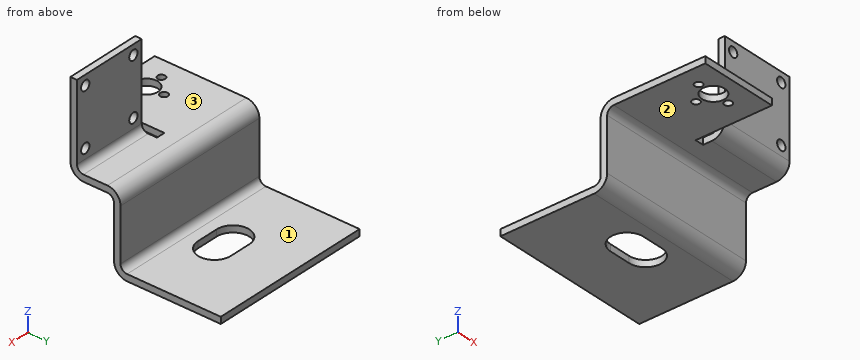
from build123d import *

# Parameters (mm, degrees)
SKETCH1_W                    = 35
SKETCH1_H                    = 35
SKETCH1_R                    = 2.25
BASE_FLANGE1_DEPTH           = 3
EDGE_FLANGE1_DEPTH           = 35
SKETCH9_W                    = 36
SKETCH9_H                    = 35
BOSS_EXTRUDE1_DEPTH          = 3
EDGE_FLANGE2_STRIP_W         = 18
EDGE_FLANGE2_STRIP_H         = 3
EDGE_FLANGE2_STRIP_CUT_DEPTH = 75
EDGE_FLANGE2_DEPTH           = 75
EDGE_FLANGE3_STRIP_W         = 18
EDGE_FLANGE3_STRIP_H         = 3
EDGE_FLANGE3_STRIP_CUT_DEPTH = 75
EDGE_FLANGE3_DEPTH           = 75
SKETCH16_R                   = 5.25
SKETCH16_R_2                 = 1.75
CUT_EXTRUDE1_DEPTH           = 10
CUT_EXTRUDE2_DEPTH           = 10
BODY_MOVE_COPY1_ANGLE        = 180


# Sheet-metal steps are written as plain solids
with BuildPart() as part:
    # Sketch1 → Base-Flange1 (new body)
    with BuildSketch(Plane.XY):
        Rectangle(SKETCH1_W, SKETCH1_H)
        with Locations((-13, 13)):
            Circle(SKETCH1_R, mode=Mode.SUBTRACT)
        with Locations((13, 13)):
            Circle(SKETCH1_R, mode=Mode.SUBTRACT)
        with Locations((13, -13)):
            Circle(SKETCH1_R, mode=Mode.SUBTRACT)
        with Locations((-13, -13)):
            Circle(SKETCH1_R, mode=Mode.SUBTRACT)
    extrude(amount=-BASE_FLANGE1_DEPTH)

    # Edge-Flange1 section (across the edge) → Edge-Flange1 (add)
    with BuildSketch(Plane(origin=(-17.5, -20.5, 0), x_dir=(0, 1, 0), z_dir=(1, 0, 0))):
        with BuildLine():
            Line((-3, 3), (-3, 17))
            Line((-3, 17), (0, 17))
            Line((0, 17), (0, 3))
            ThreePointArc((0, 3), (0.878679656, 0.878679656), (3, 0))
            Line((3, 0), (3, -3))
            ThreePointArc((3, -3), (-1.242640687, -1.242640687), (-3, 3))
        make_face()
    extrude(amount=EDGE_FLANGE1_DEPTH)

    # Sketch9 → Boss-Extrude1 (add)
    with BuildSketch(Plane.XZ.offset(23.5)):
        Polygon((57.5, 17), (17.5, 17), (17.5, 7), (21.5, 7), (57.5, 7), align=None)
        with Locations((39.5, -10.5)):
            Rectangle(SKETCH9_W, SKETCH9_H)
    extrude(amount=-BOSS_EXTRUDE1_DEPTH)

    # Edge-Flange2 strip (across the edge) → Edge-Flange2 strip cut (cut)
    with BuildSketch(Plane(origin=(57.5, -23.5, 17), x_dir=(0, 0, -1), z_dir=(-1, 0, 0))):
        with Locations((-6, -1.5)):
            Rectangle(EDGE_FLANGE2_STRIP_W, EDGE_FLANGE2_STRIP_H)
    extrude(amount=EDGE_FLANGE2_STRIP_CUT_DEPTH, mode=Mode.SUBTRACT)

    # Edge-Flange2 section (across the edge) → Edge-Flange2 (add)
    with BuildSketch(Plane(origin=(57.5, -23.5, 17), x_dir=(0, 0, -1), z_dir=(-1, 0, 0))):
        with BuildLine():
            Line((-3, 3), (-3, 30))
            Line((-3, 30), (0, 30))
            Line((0, 30), (0, 3))
            ThreePointArc((0, 3), (0.878679656, 0.878679656), (3, 0))
            Line((3, 0), (3, -3))
            ThreePointArc((3, -3), (-1.242640687, -1.242640687), (-3, 3))
        make_face()
    extrude(amount=EDGE_FLANGE2_DEPTH)

    # Edge-Flange3 strip (across the edge) → Edge-Flange3 strip cut (cut)
    with BuildSketch(Plane(origin=(-17.5, -53.5, 20), x_dir=(0, 1, 0), z_dir=(1, 0, 0))):
        with Locations((-6, -1.5)):
            Rectangle(EDGE_FLANGE3_STRIP_W, EDGE_FLANGE3_STRIP_H)
    extrude(amount=EDGE_FLANGE3_STRIP_CUT_DEPTH, mode=Mode.SUBTRACT)

    # Edge-Flange3 section (across the edge) → Edge-Flange3 (add)
    with BuildSketch(Plane(origin=(-17.5, -53.5, 20), x_dir=(0, 1, 0), z_dir=(1, 0, 0))):
        with BuildLine():
            Line((-3, 3), (-3, 46))
            Line((-3, 46), (0, 46))
            Line((0, 46), (0, 3))
            ThreePointArc((0, 3), (0.878679656, 0.878679656), (3, 0))
            Line((3, 0), (3, -3))
            ThreePointArc((3, -3), (-1.242640687, -1.242640687), (-3, 3))
        make_face()
    extrude(amount=EDGE_FLANGE3_DEPTH)

    # Sketch16 → Cut-Extrude1 (cut)
    with BuildSketch(Plane(origin=(0, -20.5, 0), x_dir=(1, 0, 0), z_dir=(0, 1, 0))):
        with Locations(Location((40.5, 17.3, 0), (0, 0, 270))):
            Circle(SKETCH16_R)
        with Locations(Location((40.5, 9.3, 0), (0, 0, 270))):
            Circle(SKETCH16_R_2)
        with Locations(Location((48.5, 17.3, 0), (0, 0, 270))):
            Circle(SKETCH16_R_2)
        with Locations(Location((32.5, 17.3, 0), (0, 0, 270))):
            Circle(SKETCH16_R_2)
    extrude(amount=-CUT_EXTRUDE1_DEPTH, mode=Mode.SUBTRACT)

    # Sketch17 → Cut-Extrude2 (cut)
    with BuildSketch(Plane(origin=(0, -53.5, 0), x_dir=(1, 0, 0), z_dir=(0, 1, 0))):
        with BuildLine():
            Line((25, -43), (15, -43))
            ThreePointArc((15, -43), (7.5, -35.5), (15, -28))
            Line((15, -28), (25, -28))
            ThreePointArc((25, -28), (32.5, -35.5), (25, -43))
        make_face()
    extrude(amount=-CUT_EXTRUDE2_DEPTH, mode=Mode.SUBTRACT)


with BuildPart() as part_1:
    # Body-Move/Copy1: moved
    add(part.part.moved(Location((0, 0, 0))).rotate(Axis((20, -19.25, 19.25), (-4.937700262163626e-15, 0.7071067811864181, 0.707106781186677)), BODY_MOVE_COPY1_ANGLE))


solid = part_1.part
Design review of the part built by this model. Coordinates are the model's own, in mm. Face numbers are marked on the shaded views. A direction names the side the tool comes from. Give positions to 0.01 mm unless a question says otherwise; leave off trailing zeros. Order: outer loops, then holes, each group sorted by start corner. A loop starts at its lowest first (then second) coordinate and runs counter-clockwise, first axis right, second up.
1. Tool access review of the marked faces 1, 2 and 3: name each direction out of +Z, -Z, +X, -X, +Y, -Y from which nothing blocks a thin tool from reaching the whole face with its end or side.
Solution:
face 1: +Z, +X, -X, +Y
face 2: -Z, +X, -X, -Y
face 3: +Z, -X, +Y
2. Add section D-D, the plane x = -8.5. State the section outline as (y, z) points, then the cut area to 3 significant figures.
Solution:
outline: (-66.5, 15) - (-57.55, 15) - (-57.55, 18) - (-66.5, 18) - close; (-54.05, 15) - (-24.5, 15) arc R3 cw to (-21.5, 12) - (-21.5, -12) arc R6 ccw to (-15.5, -18) - (27.5, -18) - (27.5, -15) - (-15.5, -15) arc R3 cw to (-18.5, -12) - (-18.5, 12) arc R6 ccw to (-24.5, 18) - (-54.05, 18) - close
area: 359 mm2
3. Add section B-B, the plane z = 51.5. State the section outline as (x, y) points.
Solution:
outline: (22.5, -41.5) - (24.75, -41.5) - (24.75, -38.5) - (22.5, -38.5) - close; (29.25, -41.5) - (50.75, -41.5) - (50.75, -38.5) - (29.25, -38.5) - close; (55.25, -41.5) - (57.5, -41.5) - (57.5, -38.5) - (55.25, -38.5) - close
4. Add section C-C, the plane y = -47.8. State the section outline as (x, z) points, then the cut area to 3 significant figures.
Solution:
outline: (-17.5, 15) - (-2.25, 15) - (-2.25, 18) - (-17.5, 18) - close; (1.25, 15) - (18.5, 15) - (18.5, 18) - (1.25, 18) - close
area: 97.5 mm2
5. To check wall thickness, follow L1, parallel to X at y = -55.8, z = 16.25; L2, parallel to X at y = -39.5, z = 25.5; L3, parallel to Y at x = 0, z = 16. State the ranges of each line that lie inside material, in increasing order.
Solution:
L1: x = -17.5 to -10.25, -6.75 to -5.75, 4.75 to 5.75, 9.25 to 18.5
L2: x = 22.5 to 24.75, 29.25 to 50.75, 55.25 to 57.5
L3: y = -66.5 to -61.03, -50.57 to -49.48, -46.12 to -20.03
6. For pin 1 Ø8 at (x, z) = (48.5, 6.5) entering from +Y; pin 2 Ø8 at (y, z) = (-34, 36) entering from -X; pin 3 Ø10.5 at (x, z) = (36, 38) entering from -Y; pin 4 Ø4 at (x, y) = (-8.5, -55.8) entering from +Z, all flat-tipped, find the tip position at first contact; note any pin that passes through.
Solution:
pin 1: stops at y = -18.5
pin 2: passes through
pin 3: stops at y = -41.5
pin 4: stops at z = 18
7. Add section A-A, the plane x = -0.5. State the section outline as (y, z) points, then the cut area to 3 significant figures.
Solution:
outline: (-66.5, 15) - (-61.05, 15) - (-61.05, 18) - (-66.5, 18) - close; (-50.55, 15) - (-49.55, 15) - (-49.55, 18) - (-50.55, 18) - close; (-46.05, 15) - (-24.5, 15) arc R3 cw to (-21.5, 12) - (-21.5, -12) arc R6 ccw to (-15.5, -18) - (27.5, -18) - (27.5, -15) - (-15.5, -15) arc R3 cw to (-18.5, -12) - (-18.5, 12) arc R6 ccw to (-24.5, 18) - (-46.05, 18) - close
area: 327 mm2
